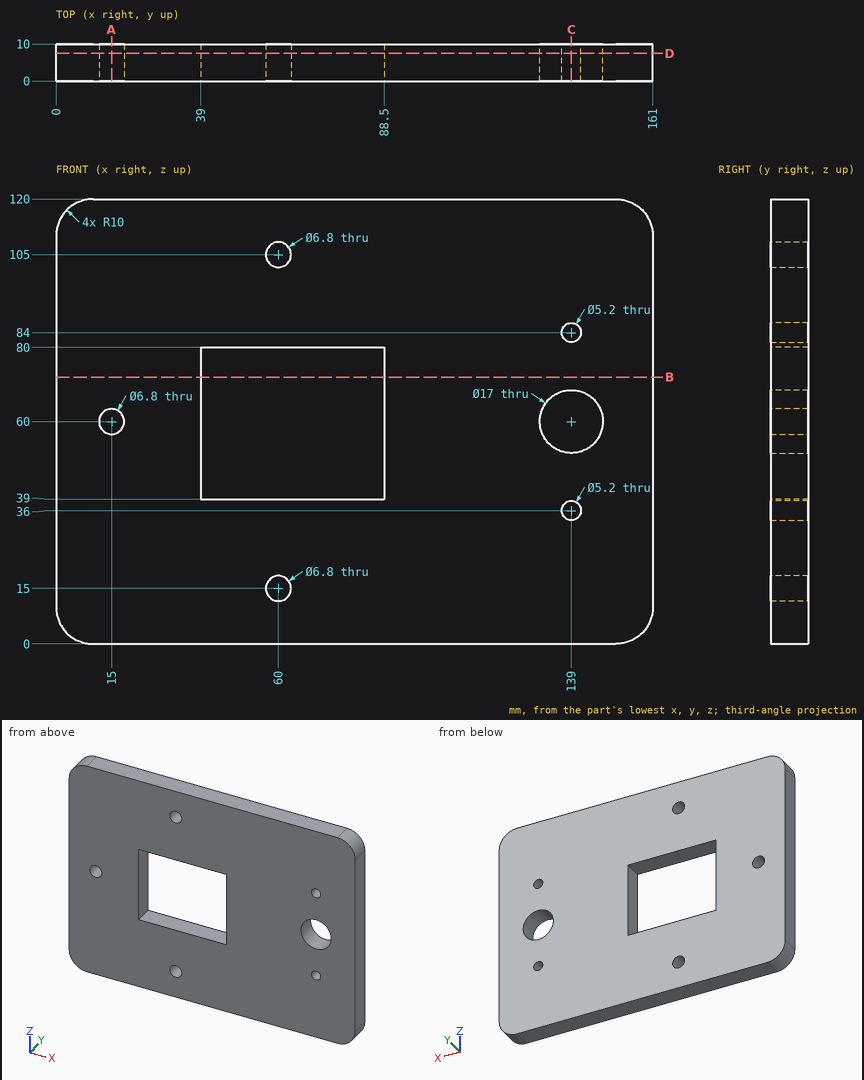
The drawing under review shows one solid part. Ordinate dimensions are in mm from its lowest x, y, z. Coordinates: 2 decimals unless noted, no trailing zeros. Write each loop counter-clockwise with the first axis right and the second up, starting at its lowest first coordinate (ties: lowest second). Pieces come first, ordered by that corner, then holes.
1) Insertion check: pin 1 (15.5 mm diameter, centred on x = 139, z = 60, fed in from +Y). The pin has a flat end and moves straight along its axis. Give the tip position at first contact, or say it passes through.
2) Add section B-B (z = 72). Write out the cut boundary in (x, y), plus the area to 4 significant figures.
3) Add section C-C (x = 139). Write out the cut boundary in (y, z), plus the area to 3 significant figures.
4) Add section D-D (y = 7.5). Write out the cut boundary in (x, z).
5) Add section A-A (x = 15). Write out the cut boundary in (y, z).
6) To check wall thickness, follow L1, parallel to X at y = 3.5, z = 70.5; L2, parallel to X at y = 7, z = 60; L3, parallel to X at y = 7.75, z = 105. State the ranges of each line that lie inside material, in increasing order.
Check result:
1. pin 1: passes through
2. outline: (0, 0) - (39, 0) - (39, 10) - (0, 10) - close; (88.5, 0) - (161, 0) - (161, 10) - (88.5, 10) - close
2. area: 1,115 mm2
3. outline: (0, 0) - (10, 0) - (10, 33.4) - (0, 33.4) - close; (0, 38.6) - (10, 38.6) - (10, 51.5) - (0, 51.5) - close; (0, 68.5) - (10, 68.5) - (10, 81.4) - (0, 81.4) - close; (0, 86.6) - (10, 86.6) - (10, 120) - (0, 120) - close
3. area: 926 mm2
4. outline: (0, 10) arc R10 ccw to (10, 0) - (151, 0) arc R10 ccw to (161, 10) - (161, 110) arc R10 ccw to (151, 120) - (10, 120) arc R10 ccw to (0, 110) - close; hole circle Ø6.8 at (15, 60); hole (39, 39) - (88.5, 39) - (88.5, 80) - (39, 80) - close; hole circle Ø6.8 at (60, 15); hole circle Ø6.8 at (60, 105); hole circle Ø17 at (139, 60); hole circle Ø5.2 at (139, 36); hole circle Ø5.2 at (139, 84)
5. outline: (0, 0) - (10, 0) - (10, 56.6) - (0, 56.6) - close; (0, 63.4) - (10, 63.4) - (10, 120) - (0, 120) - close
6. L1: x = 0 to 39, 88.5 to 161
6. L2: x = 0 to 11.6, 18.4 to 39, 88.5 to 130.5, 147.5 to 161
6. L3: x = 0 to 56.6, 63.4 to 161
